```python
from build123d import *

# Parameters (mm, degrees)
FILLET1_R          = 4
SKETCH3_R          = 4
CUT_EXTRUDE1_DEPTH = 42.546660516


with BuildPart() as part:
    # Sketch1 → Revolve1 (revolve)
    with BuildSketch(Plane(origin=(0, 0, 0), x_dir=(-1, 0, 0), z_dir=(0, 1, 0)), mode=Mode.PRIVATE) as revolve1_sk:
        Polygon((-10, 0), (-10, 25.75), (-6, 25.75), (-6, 15.25), (6, 15.25), (6, 25.75), (10, 25.75), (10, 0), align=None)
    revolve(revolve1_sk.sketch.rotate(Axis((10, 0, 0), (-1, 0, 0)), 180), axis=Axis((10, 0, 0), (-1, 0, 0)))

    # Fillet1
    fillet1_edges = [part.edges().sort_by_distance(p)[0] for p in [
        (6, 0, 15.25),
        (-6, 0, 15.25),
    ]]
    fillet(fillet1_edges, radius=FILLET1_R)

    # Sketch3 → Cut-Extrude1 (cut, through all)
    with BuildSketch(Plane(origin=(-10, 0, 0), x_dir=(0, -1, 0), z_dir=(-1, 0, 0))):
        with Locations(Location((0, 0, 0), (0, 0, 90))):
            Circle(SKETCH3_R)
    extrude(amount=-CUT_EXTRUDE1_DEPTH, mode=Mode.SUBTRACT)


solid = part.part
```
Can you work these out from the model? Positions are in its coordinate system, mm. A direction names the side the tool comes from. Coordinates: 2 decimals unless noted, no trailing zeros. Loops run counter-clockwise (first coordinate to the right, second up) from the corner with the lowest first, then second, coordinate; pieces in that order, holes last. Notation, with made-up numbers: (-3.5, 50) -> (3.5, 50) arc R24 cw to (3.5, 80) -> close; hole circle Ø4 at (-33, 84). An arc over 180 degrees is marked (long way). Put each result on its own line as item: value. Start each with the question number.
Q1. I'm going to push flat-ended pins straight in: P1, Ø10, axis at x = 1.5, y = 15, coming from the +Z side; P2, Ø3, axis at x = -1.5, y = 4, coming from the +Z side; P3, Ø2, axis at x = 1.5, z = 4, coming from the +Y side. Where does each tip first touch, or does it pass through?
Q2. I want a section at C-C (x = 0.25). Write out the boundary of the cut face in (y, z).
Q3. If I drill on line 1 (Y direction, x = -1.75, z = 0); line 2 (X direction, y = -23, z = 0); line 3 (Y direction, x = -3, z = 0), over which ranges is the centre line in solid material (lowest first)? Write a range as [from, to].
Q4. I want a section at D-D (z = 21.5). Write out the boundary of the cut face in (x, y).
Q5. Thinking about a two-plate mould opening in X: for faces 3 (the face through (6, 19, -4)), 4 (the face through (-10, 5, 0)), 5 (the face through (10, 0, 5)), which applies, pulls with the +X half, pulls with the -X half, needs draft (parallel to the pull), parting line crosses it, or undercut?
Q6. I want a section at A-A (y = 0). Write out the boundary of the cut face in (x, z).
Q7. For faces 1 (the face through (-8.028, 22.845, -11.882)), 2 (the face through (-6, 19, 4)), which set-ups out of +Z, -Z, +X, -X, +Y, -Y let a thin tool reach every point of the face, with its end or its side?
Taken from the geometry:
1. P1: stops at z = 22.33
1. P2: stops at z = 15.04
1. P3: stops at y = 14.95
2. outline: circle Ø30.5 at (0, 0); hole circle Ø8 at (0, 0)
3. line 1: y = [-15.25, -4], [4, 15.25]
3. line 2: x = [-10, -6], [6, 10]
3. line 3: y = [-15.38, -4], [4, 15.38]
4. outline: (-10, -14.17) -> (-6, -14.17) -> (-6, 14.17) -> (-10, 14.17) -> close; (6, -14.17) -> (10, -14.17) -> (10, 14.17) -> (6, 14.17) -> close
5. face 3: undercut
5. face 4: pulls with the -X half
5. face 5: pulls with the +X half
6. outline: (-10, -25.75) -> (-6, -25.75) -> (-6, -19.25) arc R4 cw to (-2, -15.25) -> (2, -15.25) arc R4 cw to (6, -19.25) -> (6, -25.75) -> (10, -25.75) -> (10, -4) -> (-10, -4) -> close; (-10, 4) -> (10, 4) -> (10, 25.75) -> (6, 25.75) -> (6, 19.25) arc R4 cw to (2, 15.25) -> (-2, 15.25) arc R4 cw to (-6, 19.25) -> (-6, 25.75) -> (-10, 25.75) -> close
7. face 1: +X, -X
7. face 2: none
